from build123d import *

# Parameters (mm, degrees)
F0_W      = 57.15
F0_H      = 44.45
F2_DEPTH  = 25.4
F3_W      = 44.45
F3_H      = 31.75
F4_DEPTH  = 25.4
F6_DEPTH  = 25.4
F8_DEPTH  = 25.4
F10_DEPTH = 25.4
F11_R     = 6.35
F12_DEPTH = 25.4


with BuildPart() as f2:
    # F0 (on Front) → F2 (new body)
    with BuildSketch(Plane.XZ):
        with Locations((28.575, 22.225)):
            Rectangle(F0_W, F0_H)
    extrude(amount=F2_DEPTH)

    # F3 (on face) → F4 (cut)
    with BuildSketch(Plane.XZ.offset(25.4)):
        with Locations((34.925, 28.575)):
            Rectangle(F3_W, F3_H)
    extrude(amount=-F4_DEPTH, mode=Mode.SUBTRACT)

    # F5 (on face) → F6 (cut)
    with BuildSketch(Plane(origin=(0, 0, 0), x_dir=(0, -1, 0), z_dir=(-1, 0, 0))):
        with BuildLine():
            ThreePointArc((0, 34.065149012), (12.5994370477, 43.9648535962), (25.4, 34.3266196875))
            Line((25.4, 34.3266196875), (25.4, 44.45))
            Line((25.4, 44.45), (0, 44.45))
            Line((0, 44.45), (0, 34.065149012))
        make_face()
    extrude(amount=-F6_DEPTH, mode=Mode.SUBTRACT)

    # F7 (on face) → F8 (cut)
    with BuildSketch(Plane(origin=(0, 0, 0), x_dir=(0, -1, 0), z_dir=(-1, 0, 0))):
        with BuildLine():
            ThreePointArc((20.7597522167, 41.230371503), (12.6668838252, 43.9653747873), (4.6026757381, 41.1469870045))
            ThreePointArc((4.6026757381, 41.1469870045), (12.7494064505, 27.9752999749), (20.7597522167, 41.230371503))
        make_face()
    extrude(amount=-F8_DEPTH, mode=Mode.SUBTRACT)

    # F9 (on face) → F10 (cut)
    with BuildSketch(Plane.XY.offset(12.7)):
        with BuildLine():
            ThreePointArc((49.7347712517, 0), (57.0352782302, -13.2327718435), (48.0707809329, -25.4))
            Line((48.0707809329, -25.4), (57.15, -25.4))
            Line((57.15, -25.4), (57.15, 0))
            Line((57.15, 0), (49.7347712517, 0))
        make_face()
    extrude(amount=-F10_DEPTH, mode=Mode.SUBTRACT)

    # F11 (on face) → F12 (cut)
    with BuildSketch(Plane.XY.offset(12.7)):
        with Locations((22.7237032021, -13.4871597779)):
            Circle(F11_R)
        with Locations((43.0526448926, -12.3167495402)):
            Circle(F11_R)
    extrude(amount=-F12_DEPTH, mode=Mode.SUBTRACT)


solid = f2.part
Part model, mm, in its own coordinate system. A direction names the side the tool comes from. Give positions to 0.01 mm unless a question says otherwise; leave off trailing zeros. Order: outer loops, then holes, each group sorted by start corner. A loop starts at its lowest first (then second) coordinate and runs counter-clockwise, first axis right, second up. Notation, with made-up numbers: (-32.5, 41.5) - (-28.5, 41.5) arc R23 ccw to (-28.5, 59.5) - close; hole circle Ø3 at (79, 7). An arc over 180 degrees is marked (long way). One line per question, with ' | ' between items.
1. Band-saw the part on B-B on x = 45. List the corners of the cut face in (y, z).
Filled in:
outline: (-25.4, 0) - (-18.36, 0) - (-18.36, 12.7) - (-25.4, 12.7) - close; (-6.27, 0) - (0, 0) - (0, 12.7) - (-6.27, 12.7) - close
2. Band-saw the part on C-C on z = 21. List the corners of the cut face in (x, y).
Filled in:
outline: (0, -25.4) - (12.7, -25.4) - (12.7, 0) - (0, 0) - close
3. Band-saw the part on D-D on x = 32.5. List the corners of the cut face in (y, z), then the cut area to 3 significant figures.
Filled in:
outline: (-25.4, 0) - (0, 0) - (0, 12.7) - (-25.4, 12.7) - close | area: 323 mm²
4. Band-saw the part on A-A on y = -8.25. List the corners of the cut face in (x, z), then the cut area to 3 significant figures.
Filled in:
outline: (0, 0) - (19.13, 0) - (19.13, 12.7) - (12.7, 12.7) - (12.7, 29.14) - (0, 29.14) - close; (26.31, 0) - (38.18, 0) - (38.18, 12.7) - (26.31, 12.7) - close; (47.93, 0) - (56.46, 0) - (56.46, 12.7) - (47.93, 12.7) - close | area: 711 mm²
5. Pull direction Z, two halves, no side cores. Call faces 3 (the face through (6.261, -12.49, 27.978)), 4 (the face through (35, -13, 12.7)), 5 (the face through (0, -13, 16)): +Z half, -Z half, draft (parallel to the pull), parting line (faces both ways), or undercut.
Filled in:
face 3: undercut | face 4: +Z half | face 5: draft
6. Drill centre lines: probe 1 along X at (y, z) = (-9, 5); probe 2 along Z at (x, y) = (53, -13.5). Where is each one in solid material? Low to high.
Filled in:
probe 1: 0 to 18.23, 27.22 to 37.64, 48.47 to 56.67 | probe 2: 0 to 12.7
7. Drop flat-ended pins along their axis: P1, Ø12.5, axis at x = 40, y = -16.5, coming from the +Z side; P2, Ø8, axis at y = -20.5, z = 36.5, coming from the +X side. Give the stop position or say it passes through.
Filled in:
P1: z = 12.7 | P2: x = 12.7
8. Which spindle directions (+Z, -Z, +X, -X, +Y, -Y) get a long thin tool onto all of the face, cutting with end or side? Do faces 1 (the face through (6.261, -1.684, 37.935)), 2 (the face through (12.7, -13, 24)). Say none if no direction does.
Filled in:
face 1: +Z, +X, -X, +Y | face 2: +Z, +X, +Y, -Y
